Verification items for this drawing (mm, ordinates from the low corner). A direction names the side the tool comes from. Coordinates: 2 decimals unless noted, no trailing zeros. Write each loop counter-clockwise with the first axis right and the second up, starting at its lowest first coordinate (ties: lowest second). Pieces come first, ordered by that corner, then holes. Notation, with made-up numbers: M -29,-22.5 L -3,-22.5 A13 cw -3,1.5 Z; hole C 15.5,56.25 d9. An arc over 180 degrees is marked long. Put each result on its own line as item: value. Start each with the question number.
1) Gauge pin test, flat end, axial feed: pin 1 (5 mm diameter, centred on x = 13.5, y = 8.5, fed in from -Z). Record the tip position at first contact, or that the pin passes through.
2) Set-up check for the marked faces 5 and 6: record each of +Z, -Z, +X, -X, +Y, -Y from which the full face is reachable in a straight line by a thin tool's end or side.
3) Cross-section at A-A on x = 3.5. Record the cut outline in (y, z) (3 decimals).
4) Cross-section at C-C on y = 7.75. Record the cut outline in (x, z) (3 decimals).
5) Cross-section at B-B on z = 4.5. Record the cut outline in (x, y), plus the area to 3 significant figures.
6) Cross-section at D-D on z = 6. Record the cut outline in (x, y).
7) Mould release check, pull along X, two halves, no side actions. Record for the marked faces 1, 2, 3 and 4: released by +X, released by -X, zero draft, split by the parting line, or undercut.
8) Scan lines: line 1 along Z through (x, y) = (3.5, 4.25) (3 decimals); line 2 along X through (y, z) = (6, 2.75); line 3 along X through (y, z) = (2.75, 4.5). Record each from-to range of solid material in increasing order.
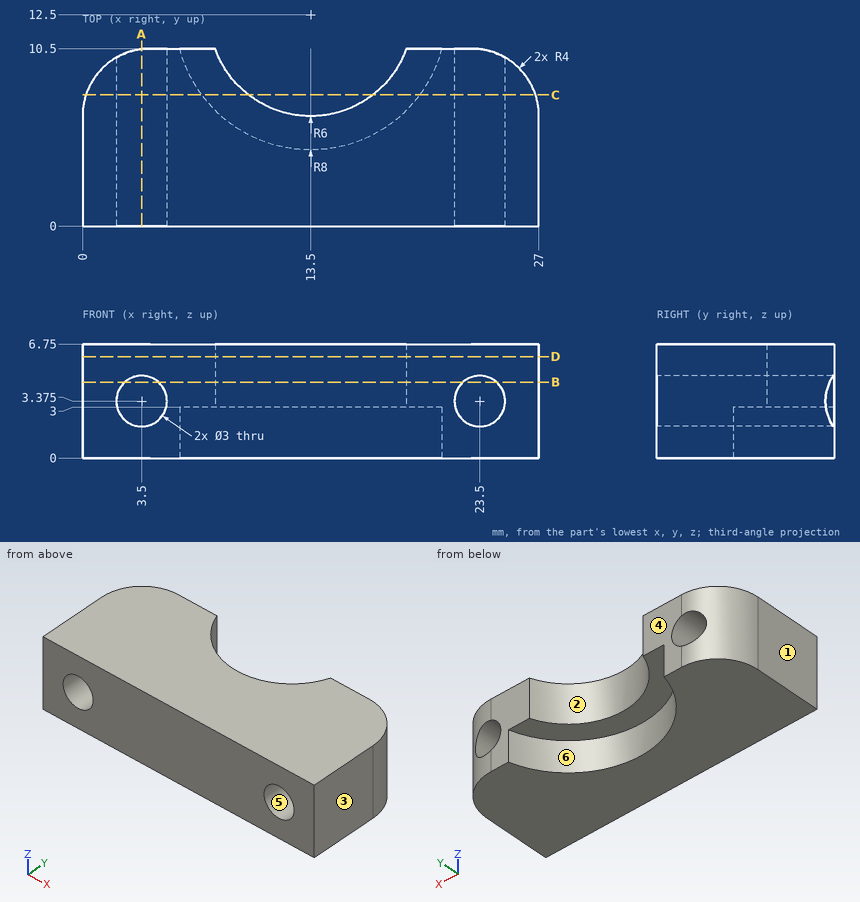
Answer key:
1. pin 1: stops at z = 3
2. face 5: +Y, -Y
2. face 6: -Z, +Y
3. outline: M 0,0 L 10.469,0 L 10.469,1.875 L 0,1.875 Z; M 0,4.875 L 10.469,4.875 L 10.469,6.75 L 0,6.75 Z
4. outline: M 0.2,0 L 7.063,0 L 7.063,3 L 9.834,3 L 9.834,6.75 L 0.2,6.75 Z; M 17.166,3 L 19.937,3 L 19.937,0 L 26.8,0 L 26.8,6.75 L 17.166,6.75 Z; hole C 3.5,3.375 d3; hole C 23.5,3.375 d3
5. outline: M 0,0 L 2.51,0 L 2.51,10.21 A4 ccw 0,6.5 Z; M 4.49,0 L 22.51,0 L 22.51,10.5 L 19.16,10.5 A6 cw 7.84,10.5 L 4.49,10.5 Z; M 24.49,0 L 27,0 L 27,6.5 A4 ccw 24.49,10.21 Z
5. area: 202 mm²
6. outline: M 0,0 L 27,0 L 27,6.5 A4 ccw 23,10.5 L 19.16,10.5 A6 cw 7.84,10.5 L 4,10.5 A4 ccw 0,6.5 Z
7. face 1: released by -X
7. face 2: undercut
7. face 3: released by +X
7. face 4: zero draft
8. line 1: z = 0 to 1.875, 4.875 to 6.75
8. line 2: x = 0 to 2.14, 4.86 to 8.84, 18.16 to 22.14, 24.86 to 27
8. line 3: x = 0 to 2.51, 4.49 to 22.51, 24.49 to 27
